The drawing under review shows one solid part. Ordinate dimensions are in mm from its lowest x, y, z. A direction names the side the tool comes from. Give positions to 0.01 mm unless a question says otherwise; leave off trailing zeros. Loops run counter-clockwise (first coordinate to the right, second up) from the corner with the lowest first, then second, coordinate; pieces in that order, holes last.
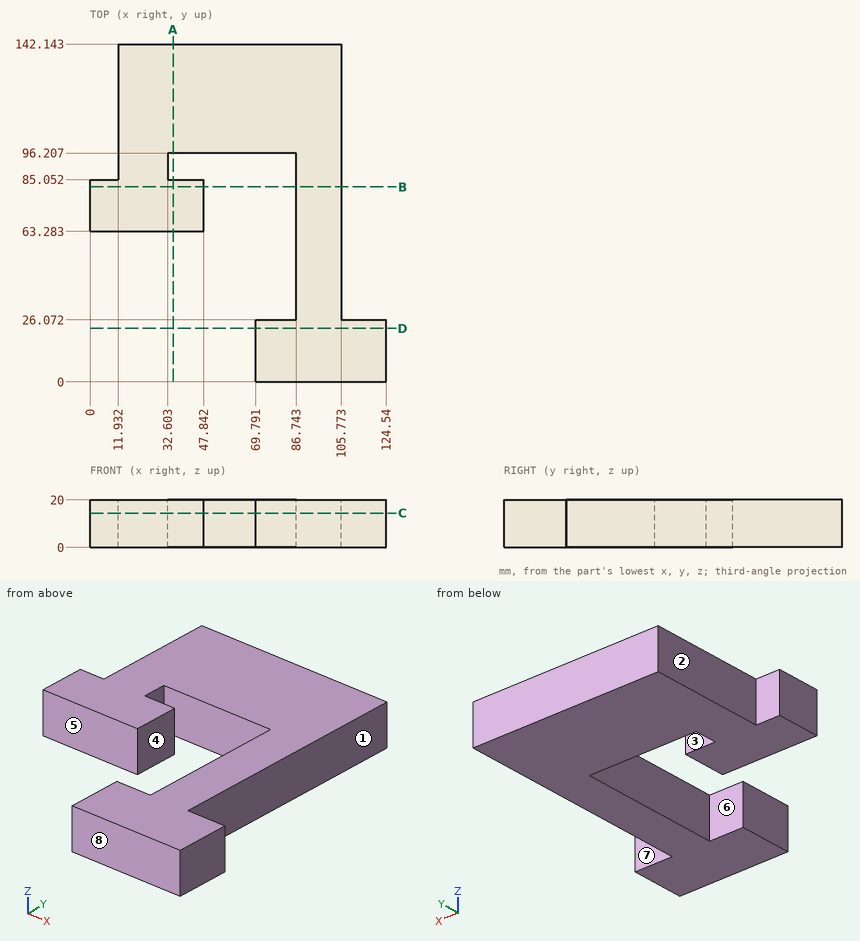
Item 1: For L1, parallel to Y at x = 74.5, z = 8.25; L2, parallel to X at y = 58.5, z = 5.5; L3, parallel to Y at x = 64, z = 14.25, list the stretches that pass through material, from the lowest coordinate up.
Answer:
L1: y = 0 to 26.07, 96.21 to 142.14
L2: x = 86.74 to 105.77
L3: y = 96.21 to 142.14
Item 2: The part is to be moulded in two halves that separate along Y. For the marked faces 6, 7 and 8, say which applies: released by +Y, released by -Y, zero draft, split by the parting line, or undercut.
Answer:
face 6: undercut
face 7: released by +Y
face 8: released by -Y
Item 3: Tool access review of the marked faces 1, 2, 3, 4 and 5: name each direction out of +Z, -Z, +X, -X, +Y, -Y from which nothing blocks a thin tool from reaching the whole face with its end or side.
Answer:
face 1: +Z, -Z, +X, +Y
face 2: +Z, -Z, -X, +Y
face 3: +Z, -Z
face 4: +Z, -Z, -Y
face 5: +Z, -Z, -X, -Y
Item 4: Take a section at B-B on y = 82. Give the boundary of the cut face in (x, z), and give its area (3 significant figures).
Answer:
outline: (0, 0) - (47.84, 0) - (47.84, 20) - (0, 20) - close; (86.74, 0) - (105.77, 0) - (105.77, 20) - (86.74, 20) - close
area: 1,340 mm2
Item 5: Clearance check with flat-ended pins moving along their axes: pin 1 Ø4 at (x, z) = (31, 9) entering from -Y; pin 2 Ø5 at (y, z) = (98, 4) entering from +X; pin 3 Ø6 at (x, z) = (63, 9.5) entering from -Y. State where each tip first meets the part, or that it passes through.
Answer:
pin 1: stops at y = 63.28
pin 2: stops at x = 105.77
pin 3: stops at y = 96.21
Item 6: Take a section at C-C on z = 14.5. Give the boundary of the cut face in (x, y).
Answer:
outline: (0, 63.28) - (47.84, 63.28) - (47.84, 85.05) - (32.6, 85.05) - (32.6, 96.21) - (86.74, 96.21) - (86.74, 26.07) - (69.79, 26.07) - (69.79, 0) - (124.54, 0) - (124.54, 26.07) - (105.77, 26.07) - (105.77, 142.14) - (11.93, 142.14) - (11.93, 85.05) - (0, 85.05) - close
Item 7: Take a section at D-D on y = 22.5. Give the boundary of the cut face in (x, z).
Answer:
outline: (69.79, 0) - (124.54, 0) - (124.54, 20) - (69.79, 20) - close
Item 8: Take a section at A-A on x = 35. Give the boundary of the cut face in (y, z).
Answer:
outline: (63.28, 0) - (85.05, 0) - (85.05, 20) - (63.28, 20) - close; (96.21, 0) - (142.14, 0) - (142.14, 20) - (96.21, 20) - close
